Part print with two shaded views. Sizes in mm from the minimum x, y, z corner. A direction names the side the tool comes from. Coordinates: 2 decimals unless noted, no trailing zeros. Loops run counter-clockwise (first coordinate to the right, second up) from the corner with the lowest first, then second, coordinate; pieces in that order, holes last. Notation, with made-up numbers: (-35, -35.75) -> (-12, -35.75) arc R25 cw to (-12, -10.75) -> close; hole circle Ø8 at (-36.75, 16.25). An arc over 180 degrees is marked (long way). One line per item, written item: value. Start each with the question number.
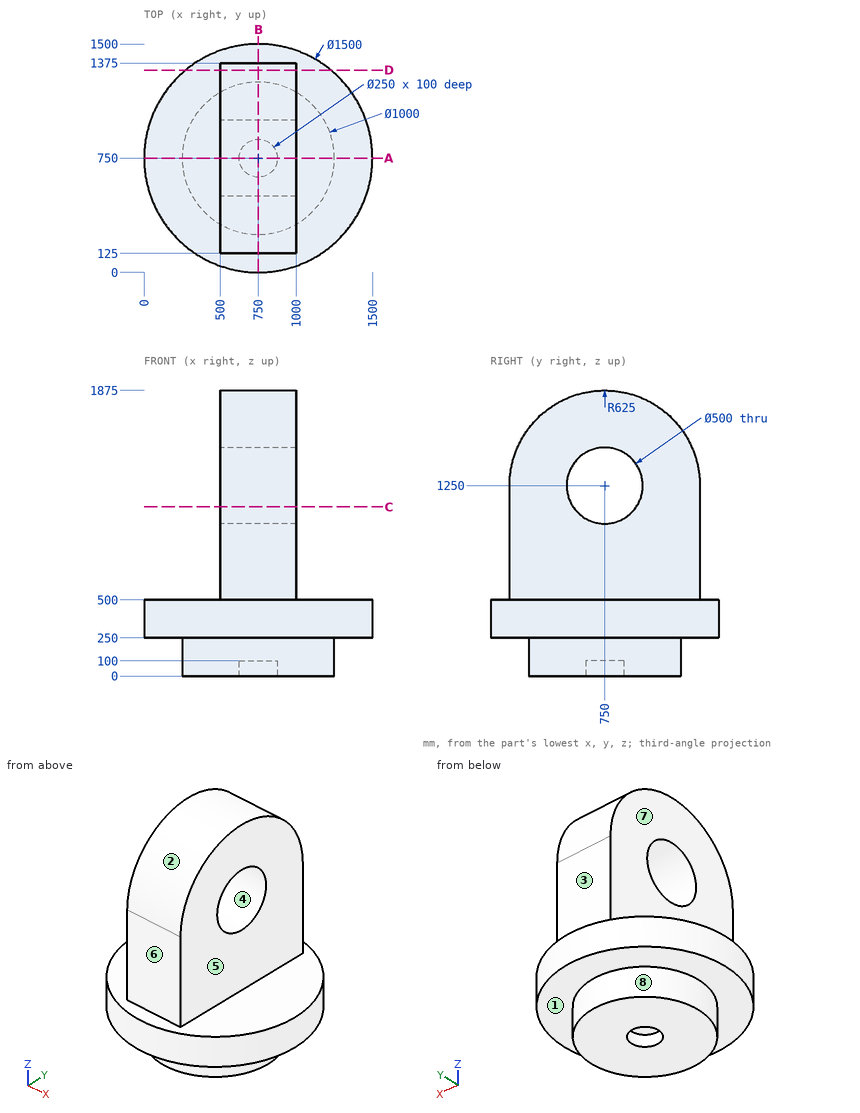
Item 1: Band-saw the part on B-B, the plane x = 750. List the corners of the cut face in (y, z).
Item 2: Band-saw the part on C-C, the plane z = 1110. List the corners of the cut face in (x, y).
Item 3: Two-plate mould, pull along Z, no slides. Class the marked faces 1, 2, 3 and 4: +Z half, -Z half, draft (parallel to the pull), parting line (faces both ways), or undercut.
Item 4: Band-saw the part on D-D, the plane y = 1328.5. List the corners of the cut face in (x, z).
Item 5: Drop flat-ended pins along their axis: pin 1 Ø4 at (y, z) = (748, 597) entering from +X; pin 2 Ø6 at (x, y) = (239, 681) entering from -Z; pin 3 Ø5 at (x, y) = (1313.5, 268.5) entering from +Z. Give the stop position or say it passes through.
Item 6: Probe probe 1 along Y at (x, z) = (750, 45); probe 2 along X at (y, z) = (612, 757.5); probe 3 along Z at (x, y) = (1341, 738). List the from-to ranges inside material, lowest first.
Item 7: Band-saw the part on A-A, the plane y = 750. List the corners of the cut face in (x, z).
Item 8: Tool access for the marked faces 5, 6, 7 and 8: list every direction of +Z, -Z, +X, -X, +Y, -Y with a clear straight run to the whole face (end or side of a thin tool).
Worked out:
1. outline: (0, 250) -> (250, 250) -> (250, 0) -> (625, 0) -> (625, 100) -> (875, 100) -> (875, 0) -> (1250, 0) -> (1250, 250) -> (1500, 250) -> (1500, 500) -> (1375, 500) -> (1375, 1250) arc R625 ccw to (125, 1250) -> (125, 500) -> (0, 500) -> close; hole circle Ø500 at (750, 1250)
2. outline: (500, 125) -> (1000, 125) -> (1000, 542.88) -> (500, 542.88) -> close; (500, 957.12) -> (1000, 957.12) -> (1000, 1375) -> (500, 1375) -> close
3. face 1: -Z half
3. face 2: +Z half
3. face 3: draft
3. face 4: undercut
4. outline: (272.68, 250) -> (1227.32, 250) -> (1227.32, 500) -> (1000, 500) -> (1000, 1486.56) -> (500, 1486.56) -> (500, 500) -> (272.68, 500) -> close
5. pin 1: stops at x = 1000
5. pin 2: stops at z = 250
5. pin 3: stops at z = 500
6. probe 1: y = 250 to 625, 875 to 1250
6. probe 2: x = 500 to 1000
6. probe 3: z = 250 to 500
7. outline: (0, 250) -> (250, 250) -> (250, 0) -> (625, 0) -> (625, 100) -> (875, 100) -> (875, 0) -> (1250, 0) -> (1250, 250) -> (1500, 250) -> (1500, 500) -> (1000, 500) -> (1000, 1000) -> (500, 1000) -> (500, 500) -> (0, 500) -> close; (500, 1500) -> (1000, 1500) -> (1000, 1875) -> (500, 1875) -> close
8. face 5: +Z, +X, +Y, -Y
8. face 6: +Z, +X, -X, -Y
8. face 7: +Z, -X, +Y, -Y
8. face 8: -Z
